Part model, mm, in its own coordinate system. Face numbers are marked on the shaded views. Give positions to 0.01 mm unless a question says otherwise; leave off trailing zeros. Order: outer loops, then holes, each group sorted by start corner. A loop starts at its lowest first (then second) coordinate and runs counter-clockwise, first axis right, second up. Notation, with made-up numbers: (3.25, 27) - (45.25, 27) arc R35 ccw to (45.25, 60) - close; hole circle Ø7 at (2.25, -1). An arc over 180 degrees is marked (long way). Use a Markdown table: item, result. Add a question column.
from build123d import *

# Parameters (mm, degrees)
BOSS_EXTRU_1_DEPTH      = 2.5
ESQUISSE2_R             = 1.2
ENL_V_MAT_EXTRU_1_DEPTH = 29.310775334
CONG_1_R                = 6
CONG_3_R                = 3
ESQUISSE4_R             = 14
ENL_V_MAT_EXTRU_2_DEPTH = 1
CONG_5_R                = 2
CHANFREIN1_SIZE         = 0.5


with BuildPart() as part:
    # Esquisse1 → Boss.-Extru.1 (new body)
    with BuildSketch(Plane(origin=(0, 0, 0), x_dir=(1, 0, 0), z_dir=(0, 1, 0))):
        with BuildLine():
            Line((-17, 22.5), (-17, -19.5))
            Line((-17, -19.5), (13.3, -19.5))
            Line((13.3, -19.5), (13.3, -8))
            Line((13.3, -8), (0, -8))
            ThreePointArc((0, -8), (-7.745966692, 2), (3.872983346, 7))
            Line((3.872983346, 7), (8.485281374, 7))
            ThreePointArc((8.485281374, 7), (3.954952524, 17.959261462), (-7, 22.5))
            Line((-7, 22.5), (-17, 22.5))
        make_face()
    extrude(amount=BOSS_EXTRU_1_DEPTH)

    # Esquisse2 → Enlèv. mat.-Extru.1 (cut, through all)
    with BuildSketch(Plane(origin=(0, 2.5, 0), x_dir=(1, 0, 0), z_dir=(0, 1, 0))):
        with Locations(Location((-14, -14, 0), (0, 0, 270))):
            Circle(ESQUISSE2_R)
        with Locations(Location((-7, 18.521339044, 0), (0, 0, 270))):
            Circle(ESQUISSE2_R)
        with Locations(Location((8, -17.5, 0), (0, 0, 270))):
            Circle(ESQUISSE2_R)
    extrude(amount=-ENL_V_MAT_EXTRU_1_DEPTH, mode=Mode.SUBTRACT)

    # Congé1
    # the kernel refuses this fillet: 6 mm, written as the material it takes off along each edge
    with BuildSketch(Plane(origin=(-17, -15, -22.5), x_dir=(0, 0, 1), z_dir=(0, 1, 0))) as cong_1_piece_1:
        with BuildLine():
            CenterArc((CONG_1_R, CONG_1_R), CONG_1_R, 180, 90)
            Line((0, CONG_1_R), (-CONG_1_R * 0.02, CONG_1_R))
            Line((-CONG_1_R * 0.02, CONG_1_R), (-CONG_1_R * 0.02, -CONG_1_R * 0.02))
            Line((-CONG_1_R * 0.02, -CONG_1_R * 0.02), (CONG_1_R, -CONG_1_R * 0.02))
            Line((CONG_1_R, -CONG_1_R * 0.02), (CONG_1_R, 0))
        make_face()
    extrude(amount=32.5, mode=Mode.SUBTRACT)
    with BuildSketch(Plane(origin=(-17, -15, 19.5), x_dir=(0, 0, -1), z_dir=(0, 1, 0)), Plane(origin=(13.3, -15, 8), x_dir=(0, 0, 1), z_dir=(0, 1, 0)), Plane(origin=(13.3, -15, 19.5), x_dir=(-1, 0, 0), z_dir=(0, 1, 0))) as cong_1_piece_2:
        with BuildLine():
            CenterArc((CONG_1_R, -CONG_1_R), CONG_1_R, 90, 90)
            Line((0, -CONG_1_R), (-CONG_1_R * 0.02, -CONG_1_R))
            Line((-CONG_1_R * 0.02, -CONG_1_R), (-CONG_1_R * 0.02, CONG_1_R * 0.02))
            Line((-CONG_1_R * 0.02, CONG_1_R * 0.02), (CONG_1_R, CONG_1_R * 0.02))
            Line((CONG_1_R, CONG_1_R * 0.02), (CONG_1_R, 0))
        make_face()
    extrude(amount=32.5, mode=Mode.SUBTRACT)
    with BuildSketch(Plane(origin=(8.485281374, -22.237247638, -7), x_dir=(-0.2862946812834453, 0, -0.9581416155604611), z_dir=(0, 1, 0))) as cong_1_piece_3:
        with BuildLine():
            CenterArc((7.171670108, 5.747215151), CONG_1_R, 192.787166877, 93.903519848)
            Line((1.320476394, 4.419234684), (1.20345252, 4.392675075))
            ThreePointArc((1.20345252, 4.392675075), (0.545261203, 2.243972704), (-0.114976994, 0.034355362))
            Line((-0.114976994, 0.034355362), (-0.034464579, -0.114944303))
            ThreePointArc((-0.034464579, -0.114944303), (4.447449528, -0.772407713), (8.929363634, -0.114944303))
            Line((8.929363634, -0.114944303), (8.894899055, 0))
        make_face()
    extrude(amount=46.974495277, mode=Mode.SUBTRACT)

    # Congé3
    cong_3_edges = [part.edges().sort_by_distance(p)[0] for p in [
        (3.872983346, 1.25, -7),
    ]]
    fillet(cong_3_edges, radius=CONG_3_R)

    # Esquisse4 → Enlèv. mat.-Extru.2 (cut)
    with BuildSketch(Plane.XZ):
        Circle(ESQUISSE4_R)
    extrude(amount=-ENL_V_MAT_EXTRU_2_DEPTH, mode=Mode.SUBTRACT)

    # Congé5
    # the kernel refuses this fillet: 2 mm, written as the material it takes off along each edge
    with BuildSketch(Plane(origin=(10.685001077, 1, 9.046035153), x_dir=(-0.696384745978129, 0, 0.7176686460818646), z_dir=(0, -1, 0))) as cong_5_piece_1:
        with BuildLine():
            CenterArc((2.033177058, -1.995401593), CONG_5_R, 93.886060886, 100.219627186)
            ThreePointArc((0.093481407, -2.482824183), (-0.083183309, -1.246303892), (0, 0))
            ThreePointArc((0, 0), (0.94881596, -0.032188852), (1.897631921, 0))
        make_face()
    extrude(amount=7.211458513, mode=Mode.SUBTRACT)
    with BuildSketch(Plane(origin=(6.925136159, 1, -12.16727123), x_dir=(-0.39164389481893525, 0, -0.9201168728216296), z_dir=(0, -1, 0))) as cong_5_piece_2:
        with BuildLine():
            CenterArc((4.592043661, -1.915459486), CONG_5_R, 73.281516472, 141.913205532)
            Line((2.957647671, -3.068173565), (2.794208072, -3.183444973))
            ThreePointArc((2.794208072, -3.183444973), (1.45226122, -1.559692524), (-0.121187489, -0.159102459))
            Line((-0.121187489, -0.159102459), (-0.080128667, 0.183246819))
            ThreePointArc((-0.080128667, 0.183246819), (3.50925175, 0.603260074), (5.224916554, 0.191545949))
            Line((5.224916554, 0.191545949), (5.167382655, 0))
        make_face()
    extrude(amount=13.918456637, mode=Mode.SUBTRACT)

    # Chanfrein1
    chanfrein1_edges = [part.edges().sort_by_distance(p)[0] for p in [
        (-14, 2.5, 12.8),
        (-7, 2.5, -19.721339044),
        (8, 2.5, 16.3),
    ]]
    chamfer(chanfrein1_edges, length=CHANFREIN1_SIZE)


solid = part.part
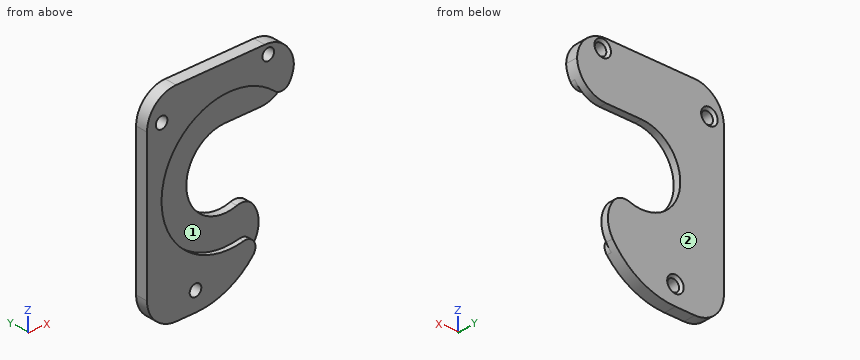
1. Mould opens along Z. For the marked faces 1 and 2 say: released by +Z, released by -Z, zero draft, split by the parting line, or undercut.
2. Cut at D-D (y = 1.4). State how many separate pieces and enclosed holes the cut face has, plus the area to 3 significant figures.
3. Drill centre lines: probe 1 along Z at (x, y) = (-6, 2.3); probe 2 along X at (y, z) = (1.4, 15); probe 3 along X at (y, z) = (2.4, -12). Where is each one in solid material? Low to high. Write a range as [from, to].
4. Cut at C-C (z = 6.5). Write the cut outline in (x, y).
5. Pin check, flat tips, straight feed: P1, Ø2, axis at x = -7, z = -18.52, coming from the -Y side; P2, Ø4, axis at x = -14, z = 14, coming from the +Y side. Stop position of each tip, or through.
6. Cut at B-B (x = -4.5). Write the cut outline in (y, z), plus the area to 3 significant figures.
7. Cut at A-A (z = 17.5). Write the cut outline in (x, y), plus the area to 3 significant figures.
Responses:
| question | item | result |
|---|---|---|
| 1 | face 1 | undercut |
| 1 | face 2 | zero draft |
| 2 | separate pieces | 1 |
| 2 | enclosed holes | 3 |
| 2 | area | 787 mm² |
| 3 | probe 1 | z = [-22.47, -19.64], [-17.4, -5.29], [5.29, 19.5] |
| 3 | probe 2 | x = [-16.81, -14.66], [-13.34, 13.11] |
| 3 | probe 3 | x = [-17, 6.92] |
| 4 | outline | (-17, 0) - (-12.4, 0) - (-12.4, 1) - (-4.66, 1) - (-4.66, 2.5) - (-17, 2.5) - close |
| 5 | P1 | passes through |
| 5 | P2 | stops at y = 2.5 |
| 6 | outline | (0, -22.3) - (2.5, -22.3) - (2.5, -6.61) - (1, -6.61) - (1, -13.26) - (0, -13.26) - close; (0, 13.26) - (1, 13.26) - (1, 6.61) - (2.5, 6.61) - (2.5, 19.5) - (0, 19.5) - close |
| 6 | area | 58.1 mm² |
| 7 | outline | (-15.47, 0) - (6.8, 0) - (6.8, 2) - (6.3, 2.5) - (-15.47, 2.5) - close; (9.2, 0) - (11.77, 0) - (11.77, 2.5) - (9.7, 2.5) - (9.2, 2) - close |
| 7 | area | 61.9 mm² |
